Source: three-view drawing plus pictorial views. Frame: mm from the lowest corner of the part. A direction names the side the tool comes from. Give positions to 0.01 mm unless a question says otherwise; leave off trailing zeros. Loops run counter-clockwise (first coordinate to the right, second up) from the corner with the lowest first, then second, coordinate; pieces in that order, holes last. Notation, with made-up numbers: (56.5, 49) -> (88.5, 49) arc R27 ccw to (88.5, 78) -> close; hole circle Ø1 at (20.25, 82). An arc over 180 degrees is marked (long way). Answer as a JSON object with one key per item and string values. Group by question number.
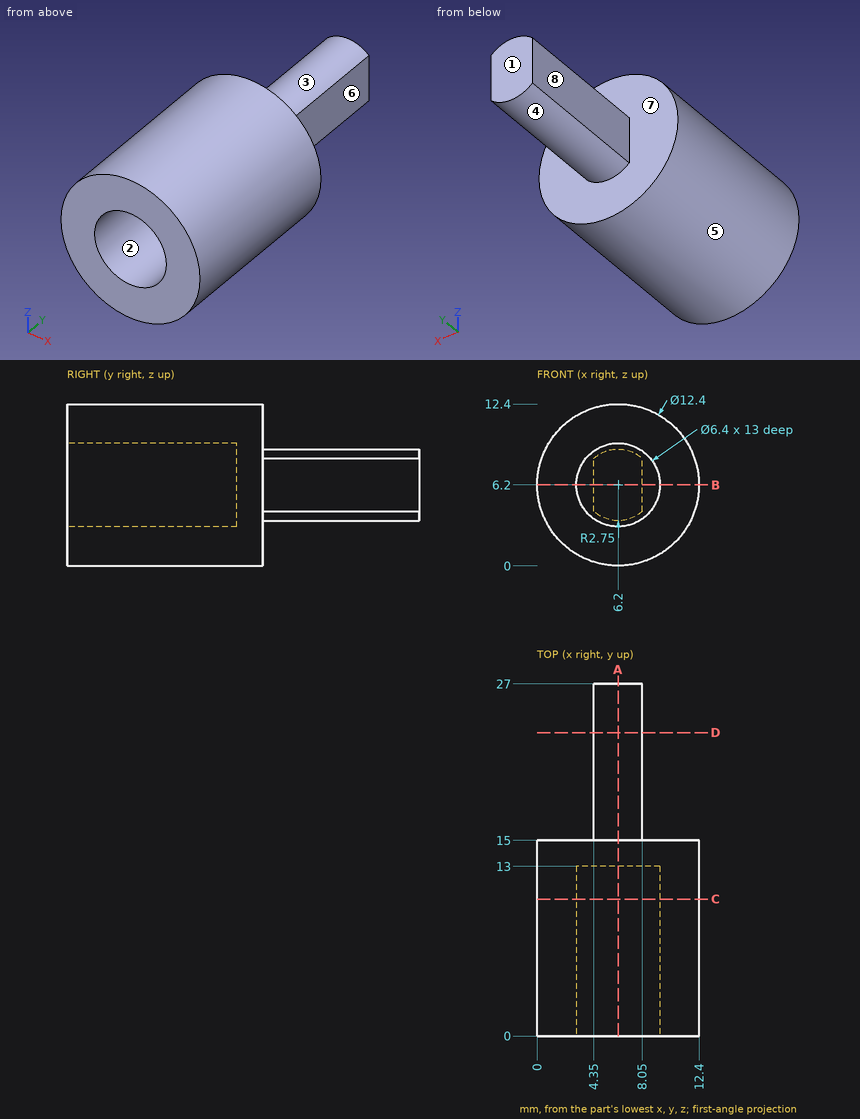
Q1. Pull-direction query (X, two-part tool) for the marked faces 1, 2 and 3; classes: +X half, -X half, draft (parallel to the pull), parting line (faces both ways), or undercut.
Q2. Pin query (flat end, axial travel): pin 1 Ø6 at (x, y) = (3, 8.5) entering from +Z; pin 2 Ø3 at (x, y) = (9, 12.5) entering from -Z; pin 3 Ø1.9 at (x, z) = (6, 5) entering from -Y. Return the tip coordinate at first contact, or that it passes through.
Q3. Section D-D on y = 23.25. Return the cut outline in (x, z).
Q4. Set-up query: the marked faces 4, 5, 6, 7 and 8. Return all of +Z, -Z, +X, -X, +Y, -Y with unobstructed straight access to the full face (end or side cutting, diameter ignored); none if empty.
Q5. Section C-C on y = 10.5. Return the cut outline in (x, z).
Q6. Section B-B on z = 6.2. Return the cut outline in (x, y), then the cut area to 3 significant figures.
Q7. Ray query, probe 1 along X at (y, z) = (7.75, 6.2); probe 2 along Z at (x, y) = (6, 3.5); probe 3 along Y at (x, z) = (8.25, 3.25). Return the intervals inside material, ascending.
Q8. Section A-A on x = 6.2. Return the cut outline in (y, z), then the cut area to 3 significant figures.
Numbers:
{
 "1": {"face 1": "draft", "face 2": "undercut", "face 3": "parting line"},
 "2": {"pin 1": "stops at z = 12.4", "pin 2": "stops at z = 0.14", "pin 3": "stops at y = 13"},
 "3": {"outline": "(4.35, 4.17) arc R2.75 ccw to (8.05, 4.17) -> (8.05, 8.23) arc R2.75 ccw to (4.35, 8.23) -> close"},
 "4": {"face 4": "-Z, +Y", "face 5": "+Y, -Y", "face 6": "+Z, -Z, +X, +Y", "face 7": "+Y", "face 8": "+Z, -Z, -X, +Y"},
 "5": {"outline": "circle Ø12.4 at (6.2, 6.2); hole circle Ø6.4 at (6.2, 6.2)"},
 "6": {"outline": "(0, 0) -> (3, 0) -> (3, 13) -> (9.4, 13) -> (9.4, 0) -> (12.4, 0) -> (12.4, 15) -> (8.05, 15) -> (8.05, 27) -> (4.35, 27) -> (4.35, 15) -> (0, 15) -> close", "area": "147 mm²"},
 "7": {"probe 1": "x = 0 to 3, 9.4 to 12.4", "probe 2": "z = 0 to 3.01, 9.39 to 12.4", "probe 3": "y = 0 to 15"},
 "8": {"outline": "(0, 0) -> (15, 0) -> (15, 3.45) -> (27, 3.45) -> (27, 8.95) -> (15, 8.95) -> (15, 12.4) -> (0, 12.4) -> (0, 9.4) -> (13, 9.4) -> (13, 3) -> (0, 3) -> close", "area": "169 mm²"}
}
